Could you check a few things on this model? Use its own coordinates, in mm. A direction names the side the tool comes from. Give positions to 0.01 mm unless a question says otherwise; leave off trailing zeros. Write each loop counter-clockwise with the first axis right and the second up, starting at its lowest first coordinate (ties: lowest second). Pieces come first, ordered by that corner, then holes. Notation, with made-up numbers: (83.25, 10) -> (121.25, 10) arc R26 ccw to (121.25, 37) -> close; hole circle Ø3 at (24, 53). An arc over 180 degrees is marked (long way). Write item = value, one per line. Start each with the question number.
Autodesk Inventor part; units mm, degrees
ref_plane "YZ Plane" through (0, 0, 0) normal (1, 0, 0) x (0, 1, 0)
ref_plane "XZ Plane" through (0, 0, 0) normal (0, 1, 0) x (-1, 0, 0)
ref_plane "XY Plane" through (0, 0, 0) normal (0, 0, 1) x (1, 0, 0)
sketch "Sketch1" plane through (0, 0, 0) normal (0, 0, 1) x (1, 0, 0)
  line L0 (8, 0) -> (-8, 0)
  line L1 (-8, 0) -> (-8, 1.6)
  line L2 (-8, 1.6) -> (0, 9.6)
  line L3 (0, 9.6) -> (8, 9.6)
  line L4 (8, 9.6) -> (8, 0)
  point P0 (0, 0)
  point P1 (0, 0)
  dimension "d0" = 9.6
  dimension "d1" = 16
  dimension "d2" = 8
  dimension "d3" = 1.6
extrude "Extrusion1" add sketch "Sketch1" along normal mid plane 16
shell "Shell1" thickness 0.8 removed faces 1 at (-2.6667, 0, 2.6667)
sketch "Sketch2" plane through (0, 9.6, 8) normal (0, 1, 0) x (1, 0, 0)
  line L0 (4, 12) -> (4, 4) construction
  line L1 (-11.2, 8) -> (11.2, 8) construction
  line L2 (8, 0) -> (8, 16) construction
  circle A0 centre (4, 12) radius 2.5
  circle A1 centre (4, 4) radius 2.5
  point P0 (4, 8)
  dimension "d6" = 4
  dimension "d7" = 8
  dimension "d8" = 5
extrude "Extrusion2" add sketch "Sketch2" along normal blind 1.6
sketch "Sketch3" plane through (0, 9.6, -8) normal (-0.7071, 0.7071, 0) x (-0.7071, -0.7071, 0)
  line L0 (11.3137, 16) -> (0, 16)
  line L1 (0, 16) -> (0, 0)
  line L2 (0, 0) -> (11.3137, 0)
  circle A0 centre (3, 2.5) radius 2
  circle A1 centre (3, 8) radius 2.5
  circle A2 centre (3, 13.5) radius 2
  line L3 (4.9365, 14) -> (6.5, 14)
  line L4 (7, 13.5) -> (7, 13.5)
  line L5 (6.5, 13) -> (4.9365, 13)
  line L6 (4.9365, 13) -> (4.9365, 14)
  line L7 (5.4495, 8.5) -> (7.013, 8.5)
  line L8 (7.513, 8) -> (7.513, 8)
  line L9 (7.013, 7.5) -> (5.4495, 7.5)
  line L10 (5.4495, 7.5) -> (5.4495, 8.5)
  line L11 (4.9365, 3) -> (6.5, 3)
  line L12 (7, 2.5) -> (7, 2.5)
  line L13 (6.5, 2) -> (4.9365, 2)
  line L14 (4.9365, 2) -> (4.9365, 3)
  arc A3 (6.5, 2) -> (7, 2.5) centre (6.5, 2.5) ccw
  arc A4 (7, 2.5) -> (6.5, 3) centre (6.5, 2.5) ccw
  arc A5 (7.013, 7.5) -> (7.513, 8) centre (7.013, 8) ccw
  arc A6 (7.513, 8) -> (7.013, 8.5) centre (7.013, 8) ccw
  arc A7 (6.5, 13) -> (7, 13.5) centre (6.5, 13.5) ccw
  arc A8 (7, 13.5) -> (6.5, 14) centre (6.5, 13.5) ccw
  point P0 (6.7882, 8)
  dimension "d12" = 4
  dimension "d13" = 5
  dimension "d14" = 4
  dimension "d15" = 5.5
  dimension "d16" = 5.5
  dimension "d17" = 2.5
  dimension "d18" = 2.5
  dimension "d19" = 3
  dimension "d20" = 0.5
  dimension "d21" = 1
  dimension "d22" = 3.5
extrude "Extrusion3" add sketch "Sketch3" along normal blind 0.01
equation "\"d14\" = d12"
equation "\"d16\" = d15"
equation "\"d17\" = d18"
properties part number "3039pc4" material "Steel"
(1) I'm going to push flat-ended pins straight in: pin 1 (3.5 mm diameter, centred on x = 3, z = -2, fed in from -Y); pin 2 (5 mm diameter, centred on y = 10, z = 1, fed in from -X); pin 3 (1 mm diameter, centred on y = 7.5, z = 5.5, fed in from -X). Where does each tip first touch, or does it pass through?
(2) Imagine slicing it at A-A (x = 1.25). Please give me the cut outline in (y, z).
(3) If I drill on line 1 along Z through (x, y) = (3.25, 0.5); line 2 along Y through (x, z) = (5.5, -1), over which ranges is the centre line in solid material (lowest first)? Write a range as from..to.
(4) Imagine slicing it at D-D (x = 4). Please give me the cut outline in (y, z).
(5) On a 3-axis mill with a long thin cutter (end or side, diameter ignored), from which of +Z, -Z, +X, -X, +Y, -Y can I reach the whole of each face in a straight line? I mean faces 1 (the flat face through (7.2, 4, 0)), 2 (the cylindrical face through (6.385, 10.389, 4.751)), 3 (the flat face through (2, 4, 8)). Say none if no direction works.
(6) Imagine slicing it at B-B (y = 2). Please give me the cut outline in (x, z).
Answers below:
q1.pin_1 = 8.8
q1.pin_2 = -2.11
q1.pin_3 = -2.61
q2.outline = (0, -8) -> (9.6, -8) -> (9.6, 8) -> (0, 8) -> (0, 7.2) -> (8.8, 7.2) -> (8.8, -7.2) -> (0, -7.2) -> close
q3.line_1 = -8..-7.2, 7.2..8
q3.line_2 = 8.8..9.6
q4.outline = (0, -8) -> (9.6, -8) -> (9.6, -6.5) -> (11.2, -6.5) -> (11.2, -1.5) -> (9.6, -1.5) -> (9.6, 1.5) -> (11.2, 1.5) -> (11.2, 6.5) -> (9.6, 6.5) -> (9.6, 8) -> (0, 8) -> (0, 7.2) -> (8.8, 7.2) -> (8.8, -7.2) -> (0, -7.2) -> close
q5.face_1 = -Y
q5.face_2 = +Y
q5.face_3 = +Z, +X, -X, +Y, -Y
q6.outline = (-7.6, -8) -> (8, -8) -> (8, 8) -> (-7.6, 8) -> close; hole (-6.47, -7.2) -> (7.2, -7.2) -> (7.2, 7.2) -> (-6.47, 7.2) -> close
